from build123d import *

# Parameters (mm, degrees)
BOSS_EXTRUDE1_DEPTH      = 27.84
SKETCH6_R                = 1.7
CUT_EXTRUDE1_DEPTH       = 13.15
SKETCH7_W                = 6
SKETCH7_H                = 2.5
CUT_EXTRUDE2_DEPTH       = 6
CHAMFER1_SIZE            = 1
CHAMFER1_OF_MIRROR2_SIZE = 1
SKETCH8_W                = 5
SKETCH8_H                = 15.8
CUT_EXTRUDE3_DEPTH       = 6.9
CUT_EXTRUDE4_REACH       = 56.65
SKETCH9_W                = 20.25
SKETCH9_H                = 10.5


with BuildPart() as part:
    # Sketch5 → Boss-Extrude1 (new body)
    with BuildSketch(Plane.XY):
        Polygon((8, 4), (8, 0), (13.9, 0), (13.9, 7.9), align=None)
        Polygon((-20.25, 27.325), (-20.25, 20.375), (0, 20.375), (0, 0), (8, 0), (8, 27.325), align=None)
    boss_extrude1 = extrude(amount=BOSS_EXTRUDE1_DEPTH)

    # Sketch6 → Cut-Extrude1 (cut)
    with BuildSketch(Plane(origin=(0, 0, 0), x_dir=(-1, 0, 0), z_dir=(0, 0, -1))):
        with Locations((4.83, 24.005)):
            Circle(SKETCH6_R)
        with Locations((15.43, 24.005)):
            Circle(SKETCH6_R)
    cut_extrude1 = extrude(amount=-CUT_EXTRUDE1_DEPTH, mode=Mode.SUBTRACT)

    # Sketch7 → Cut-Extrude2 (cut)
    with BuildSketch(Plane(origin=(0, 27.325, 0), x_dir=(1, 0, 0), z_dir=(0, 1, 0))):
        with Locations((-4.83, -11.9)):
            Rectangle(SKETCH7_W, SKETCH7_H)
        with Locations((-15.43, -11.9)):
            Rectangle(SKETCH7_W, SKETCH7_H)
    cut_extrude2 = extrude(amount=-CUT_EXTRUDE2_DEPTH, mode=Mode.SUBTRACT)

    # Chamfer1
    chamfer1_edges = [part.edges().sort_by_distance(p)[0] for p in [
        (-20.25, 20.375, 13.92),
        (-20.25, 27.325, 13.92),
        (8, 27.325, 13.92),
    ]]
    chamfer(chamfer1_edges, length=CHAMFER1_SIZE)

    # Mirror2: Boss-Extrude1, Cut-Extrude1, Cut-Extrude2 across plane
    add(boss_extrude1.mirror(Plane(origin=(0, 0, 27.84), x_dir=(0, 0, 1), z_dir=(0, -1, 0))))
    add(cut_extrude1.mirror(Plane(origin=(0, 0, 27.84), x_dir=(0, 0, 1), z_dir=(0, -1, 0))), mode=Mode.SUBTRACT)
    add(cut_extrude2.mirror(Plane(origin=(0, 0, 27.84), x_dir=(0, 0, 1), z_dir=(0, -1, 0))), mode=Mode.SUBTRACT)

    # Chamfer1 of Mirror2
    chamfer1_of_mirror2_edges = [part.edges().sort_by_distance(p)[0] for p in [
        (-20.25, -20.375, 13.92),
        (-20.25, -27.325, 13.92),
        (8, -27.325, 13.92),
    ]]
    chamfer(chamfer1_of_mirror2_edges, length=CHAMFER1_OF_MIRROR2_SIZE)

    # Sketch8 → Cut-Extrude3 (cut, through all)
    with BuildSketch(Plane(origin=(8, 0, 0), x_dir=(0, 0, -1), z_dir=(1, 0, 0))):
        with Locations((-25.34, 0)):
            Rectangle(SKETCH8_W, SKETCH8_H)
    extrude(amount=CUT_EXTRUDE3_DEPTH, mode=Mode.SUBTRACT)

    # Sketch9 → Cut-Extrude4 (cut, up to next)
    with BuildSketch(Plane(origin=(0, 27.325, 0), x_dir=(1, 0, 0), z_dir=(0, 1, 0)), mode=Mode.PRIVATE) as cut_extrude4_sk1:
        with Locations((-10.125, -22.59)):
            Rectangle(SKETCH9_W, SKETCH9_H)
    cut_extrude4_tool1 = extrude(cut_extrude4_sk1.sketch, amount=-CUT_EXTRUDE4_REACH, mode=Mode.PRIVATE) & part.part
    add(cut_extrude4_tool1.solids().sort_by_distance((-10.125, 27.325, 22.59))[0], mode=Mode.SUBTRACT)


solid = part.part
Could you check a few things on this model? Use its own coordinates, in mm. A direction names the side the tool comes from. Give positions to 0.01 mm unless a question says otherwise; leave off trailing zeros. Order: outer loops, then holes, each group sorted by start corner. A loop starts at its lowest first (then second) coordinate and runs counter-clockwise, first axis right, second up. Notation, with made-up numbers: (70.25, 44.25) -> (98.25, 44.25) arc R11 ccw to (98.25, 59.25) -> close; hole circle Ø2 at (55.5, -34). An arc over 180 degrees is marked (long way). Return JSON: item names as keys, results as strings.
1. Imagine slicing it at C-C on z = 2.5. List the corners of the cut face in (x, y) for me (3 decimals), then the cut area to 3 significant figures.
Answer list:
{"outline": "(-20.25, -26.325) -> (-19.25, -27.325) -> (7, -27.325) -> (8, -26.325) -> (8, -4) -> (13.9, -7.9) -> (13.9, 7.9) -> (8, 4) -> (8, 26.325) -> (7, 27.325) -> (-19.25, 27.325) -> (-20.25, 26.325) -> (-20.25, 21.375) -> (-19.25, 20.375) -> (0, 20.375) -> (0, -20.375) -> (-19.25, -20.375) -> (-20.25, -21.375) -> close; hole circle Ø3.4 at (-15.43, -24.005); hole circle Ø3.4 at (-15.43, 24.005); hole circle Ø3.4 at (-4.83, -24.005); hole circle Ø3.4 at (-4.83, 24.005)", "area": "750 mm2"}
2. Thinking about a two-plate mould opening in Y: for faces 6 (the flat face through (-18.43, -24, 12)), 7 (the flat face through (-15, -21.325, 12)), 8 (the flat face through (-10, -20.375, 14)), which applies, pulls with the +Y half, pulls with the -Y half, needs draft (parallel to the pull), parting line crosses it, or undercut?
Answer list:
{"face 6": "needs draft", "face 7": "pulls with the -Y half", "face 8": "undercut"}
3. Imagine slicing it at D-D on y = -8.5. List the corners of the cut face in (x, z) for me.
Answer list:
{"outline": "(0, 0) -> (8, 0) -> (8, 27.84) -> (0, 27.84) -> close"}
4. On a 3-axis mill with a long thin cutter (end or side, diameter ignored), from which of +Z, -Z, +X, -X, +Y, -Y can I reach the whole of each face in a straight line? I mean faces 1 (the flat face through (12, 0, 22.84)), 2 (the flat face through (-10, 20.375, 9)), 3 (the flat face through (-6, -26, 10.65)), 4 (the flat face through (1, -6, 27.84)), 5 (the flat face through (-5, 21.325, 12)). Say none if no direction works.
Answer list:
{"face 1": "+Z, +X, +Y, -Y", "face 2": "+Z, -Z, -X", "face 3": "-Y", "face 4": "+Z, +X, -X, +Y, -Y", "face 5": "+Y"}
5. I need wall thicknesses on line 1 (Y direction, x = -4.83, z = 3) (3 decimals); line 2 (X direction, y = -24, z = 8.5); line 3 (X direction, y = -22.5, z = 1.75). Which ranges of each line are inside material? Lowest first, please. Write a range as from..to.
Answer list:
{"line 1": "y = -27.325..-25.705, -22.305..-20.375, 20.375..22.305, 25.705..27.325", "line 2": "x = -20.25..-17.13, -13.73..-6.53, -3.13..8", "line 3": "x = -20.25..-16.22, -14.64..-5.62, -4.04..8"}
6. Imagine slicing it at B-B on x = -4.83. List the corners of the cut face in (y, z) for me (3 decimals).
Answer list:
{"outline": "(-27.325, 0) -> (-25.705, 0) -> (-25.705, 10.65) -> (-27.325, 10.65) -> close; (-27.325, 13.15) -> (-21.325, 13.15) -> (-21.325, 10.65) -> (-22.305, 10.65) -> (-22.305, 0) -> (-20.375, 0) -> (-20.375, 27.84) -> (-27.325, 27.84) -> close; (20.375, 0) -> (22.305, 0) -> (22.305, 10.65) -> (21.325, 10.65) -> (21.325, 13.15) -> (27.325, 13.15) -> (27.325, 17.34) -> (20.375, 17.34) -> close; (25.705, 0) -> (27.325, 0) -> (27.325, 10.65) -> (25.705, 10.65) -> close"}
7. For pin 1 Ø3 at (x, z) = (-2.5, 20.5) entering from +Y (3 decimals); pin 2 Ø10 at (x, y) = (-10, -15) entering from +Z; pin 3 Ø3 at (y, z) = (-24, 12) entering from +X; pin 4 Ø1.8 at (x, y) = (10, -2) entering from +Z, each with a flat end and sliding along its axis, tell me the tip position at first contact or that it passes through.
Answer list:
{"pin 1": "stops at y = -20.375", "pin 2": "passes through", "pin 3": "stops at x = 8", "pin 4": "stops at z = 22.84"}
